Could you check a few things on this model? Use its own coordinates, in mm. Face numbers are marked on the shaded views. Round coordinates to 2 decimals unless told otherwise and drop trailing zeros. Write each loop counter-clockwise with the first axis right and the second up, starting at its lowest first coordinate (ties: lowest second). Pieces come first, ordered by that corner, then holes. Notation, with made-up numbers: (25, -27) - (37, -27) arc R34 cw to (37, 9) - close; hole circle Ø2 at (43, 70.5). An arc over 180 degrees is marked (long way). Write each question's results on one line, items separated by ' | '. Start each with the question number.
(1) Imagine slicing it at A-A on y = 17. Write out the boundary of the cut face in (x, z), then the cut area to 3 significant figures.
(2) Imagine slicing it at C-C on x = -12. Write out the boundary of the cut face in (y, z), then the cut area to 3 significant figures.
(3) For P1, Ø3, axis at x = -16.5, y = 4.5, coming from the -Z side; P2, Ø2.5, axis at x = 18.49, y = -14.99, coming from the +Z side; P3, Ø11.5, axis at x = 6.5, y = 6, coming from the +Z side; P4, Ø0.9, axis at x = -22, z = 16.5, coming from the -Y side, each with a flat end and sliding along its axis, tell me the tip position at first contact or that it passes through.
(4) Imagine slicing it at D-D on y = -2.5. Write out the boundary of the cut face in (x, z).
(5) Thinking about a two-plate mould opening in Z: for the marked faces 1, 2 and 3, which applies, +Z half, -Z half, draft (parallel to the pull), parting line (faces both ways), or undercut?
(6) Imagine slicing it at B-B on z = 9.75. Write out the boundary of the cut face in (x, y), then the cut area to 3 significant figures.
(7) Please list where these lines run through material, in increasing order: line 1 (X direction, y = -4, z = 13); line 2 (Y direction, x = -17, z = 3); line 3 (Z direction, x = -7, y = 7). Write a range as [from, to].
```python
from build123d import *

# Parameters (mm, degrees)
SKETCH_W      = 47
SKETCH_H      = 40
SKETCH_R      = 2
PAD_DEPTH     = 2
PAD001_DEPTH  = 14
SKETCH002_W   = 3
SKETCH002_H   = 20
PAD002_DEPTH  = 2
FILLET_R      = 1
FILLET001_R   = 1
CHAMFER_ANGLE = 45
CHAMFER_SIZE  = 1


with BuildPart() as part:
    # Sketch → Pad (new body)
    with BuildSketch(Plane.XY):
        Rectangle(SKETCH_W, SKETCH_H)
        with Locations((-18.485281, -14.985281)):
            Circle(SKETCH_R, mode=Mode.SUBTRACT)
        with Locations((18.485281, -14.985281)):
            Circle(SKETCH_R, mode=Mode.SUBTRACT)
    extrude(amount=PAD_DEPTH)

    # Sketch001 (on Face8 of Pad) → Pad001 (join)
    with BuildSketch(Plane.XY.offset(2)):
        Polygon((-23.5, -20), (23.5, -20), (23.5, 20), (22, 20), (22, -18.5), (-22, -18.5), (-22, 20), (-23.5, 20), align=None)
    extrude(amount=PAD001_DEPTH)

    # Sketch002 (on Face14 of Pad001) → Pad002 (join)
    with BuildSketch(Plane.XY.offset(16)):
        with Locations((-22, 10)):
            Rectangle(SKETCH002_W, SKETCH002_H)
        with Locations((22, 10)):
            Rectangle(SKETCH002_W, SKETCH002_H)
    extrude(amount=PAD002_DEPTH)

    # Fillet
    fillet_edges = [part.edges().sort_by_distance(p)[0] for p in [
        (22, 10, 16),
    ]]
    fillet(fillet_edges, radius=FILLET_R)

    # Fillet001
    fillet001_edges = [part.edges().sort_by_distance(p)[0] for p in [
        (-22, 10, 16),
    ]]
    fillet(fillet001_edges, radius=FILLET001_R)

    # Chamfer
    chamfer_edges = [part.edges().sort_by_distance(p)[0] for p in [
        (16.485281, -14.985281, 2),
        (-20.485281, -14.985281, 2),
    ]]
    chamfer_side = part.faces().sort_by_distance((0, 0.98697, 2))[0]
    chamfer(chamfer_edges, length=CHAMFER_SIZE, angle=CHAMFER_ANGLE, reference=chamfer_side)


solid = part.part
```
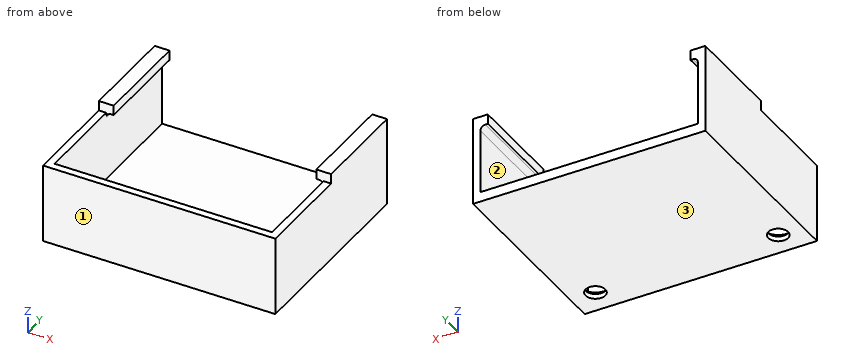
Response:
1) outline: (-23.5, 0) - (23.5, 0) - (23.5, 18) - (20.5, 18) - (20.5, 16) - (21, 16) arc R1 cw to (22, 15) - (22, 2) - (-22, 2) - (-22, 15) arc R1 cw to (-21, 16) - (-20.5, 16) - (-20.5, 18) - (-23.5, 18) - close | area: 148 mm²
2) outline: (-20, 0) - (20, 0) - (20, 2) - (-18.5, 2) - (-18.5, 16) - (-20, 16) - close | area: 101 mm²
3) P1: z = 0 | P2: through | P3: z = 2 | P4: y = 0
4) outline: (-23.5, 0) - (23.5, 0) - (23.5, 16) - (22, 16) - (22, 2) - (-22, 2) - (-22, 16) - (-23.5, 16) - close
5) face 1: draft | face 2: undercut | face 3: -Z half
6) outline: (-23.5, -20) - (23.5, -20) - (23.5, 20) - (22, 20) - (22, -18.5) - (-22, -18.5) - (-22, 20) - (-23.5, 20) - close | area: 186 mm²
7) line 1: [-23.5, -22], [22, 23.5] | line 2: [-20, -18.5] | line 3: [0, 2]
